For this review, take the finished solid that the model builds, in its own axes (mm). Face numbers are marked on the shaded views. A direction names the side the tool comes from. Coordinates: 2 decimals unless noted, no trailing zeros. Use a Markdown table: item, result.
from build123d import *

# Parameters (mm, degrees)
BASPROSKE_W        = 30
BASPROSKE_H        = 50
TOOTHCUT_DEPTH     = 77.811457479
TEETHCUTS_COUNT    = 23
TEETHCUTS_ANGLE    = 344.347826087
HUBNEABOTSKE_R     = 20
HUBNEARBOTH_DEPTH  = 5.0000254
HUBFAR_START       = 5.0000254
HUBFARSKE_R        = 20
HUBFAR_DEPTH       = 5.0000254
BORSKE_R           = 12
BORE_DEPTH         = 40.0000508
KEYSKE_W           = 8
KEYSKE_H           = 15.3
KEYWAY_DEPTH       = 40.0000508
SKETCH1_R          = 35
SKETCH1_R_2        = 20
CUT_EXTRUDE1_DEPTH = 14
FILLET1_R          = 4
CUT_EXTRUDE2_START = -14
SKETCH2_R          = 35
SKETCH2_R_2        = 20
CUT_EXTRUDE2_DEPTH = 14
FILLET2_R          = 4


with BuildPart() as part:
    # BasProSke → Base-Revolve (revolve)
    with BuildSketch(Plane(origin=(0, 0, 0), x_dir=(1, 0, 0), z_dir=(0, 1, 0)), mode=Mode.PRIVATE) as base_revolve_sk:
        with Locations((15, 25)):
            Rectangle(BASPROSKE_W, BASPROSKE_H)
    revolve(base_revolve_sk.sketch.rotate(Axis((-10, 0, 0), (1, 0, 0)), 180), axis=Axis((-10, 0, 0), (1, 0, 0)))

    # TooCutSke → ToothCut (cut, through all)
    with BuildSketch(Plane(origin=(0, 0, 0), x_dir=(0, 0, -1), z_dir=(1, 0, 0))):
        with BuildLine():
            ThreePointArc((1.90971626, 40.954498957), (0, 40.999), (-1.90971626, 40.954498957))
            ThreePointArc((-1.90971626, 40.954498957), (-3.228022445, 45.57670564), (-5.698439072, 49.699783071))
            ThreePointArc((-5.698439072, 49.699783071), (0, 50.0254), (5.698439072, 49.699783071))
            ThreePointArc((5.698439072, 49.699783071), (3.228022445, 45.57670564), (1.90971626, 40.954498957))
        make_face()
    toothcut = extrude(amount=TOOTHCUT_DEPTH, mode=Mode.SUBTRACT)

    # TeethCuts: ToothCut ×23 about axis
    teethcuts_axis = Axis((-10, 0, 0), (1, 0, 0))
    for i in range(1, TEETHCUTS_COUNT):
        add(toothcut.rotate(teethcuts_axis, i * TEETHCUTS_ANGLE / (TEETHCUTS_COUNT - 1)), mode=Mode.SUBTRACT)

    # HubNeaBotSke → HubNearBoth (add)
    with BuildSketch(Plane.ZY):
        with Locations(Location((0, 0, 0), (0, 0, 180))):
            Circle(HUBNEABOTSKE_R)
    extrude(amount=HUBNEARBOTH_DEPTH)

    # HubFarSke → HubFar (add)
    with BuildSketch(Plane(origin=(30, 0, 0), x_dir=(0, 0, -1), z_dir=(1, 0, 0)).offset(HUBFAR_START)):
        Circle(HUBFARSKE_R)
    extrude(amount=-HUBFAR_DEPTH)

    # BorSke → Bore (cut, symmetric)
    with BuildSketch(Plane(origin=(0, 0, 0), x_dir=(0, 0, -1), z_dir=(1, 0, 0))):
        with Locations(Location((0, 0, 0), (0, 0, 180))):
            Circle(BORSKE_R)
    extrude(amount=BORE_DEPTH, both=True, mode=Mode.SUBTRACT)

    # KeySke → Keyway (cut, symmetric)
    with BuildSketch(Plane(origin=(0, 0, 0), x_dir=(0, 0, -1), z_dir=(1, 0, 0))):
        with Locations((0, 7.65)):
            Rectangle(KEYSKE_W, KEYSKE_H)
    extrude(amount=KEYWAY_DEPTH, both=True, mode=Mode.SUBTRACT)

    # Sketch1 → Cut-Extrude1 (cut)
    with BuildSketch(Plane(origin=(30, 0, 0), x_dir=(0, 0, -1), z_dir=(1, 0, 0))):
        with Locations((0, 0.98088297)):
            Circle(SKETCH1_R)
        Circle(SKETCH1_R_2, mode=Mode.SUBTRACT)
    extrude(amount=-CUT_EXTRUDE1_DEPTH, mode=Mode.SUBTRACT)

    # Fillet1
    fillet1_edges = [part.edges().sort_by_distance(p)[0] for p in [
        (16, 0.98088297, 35),
        (16, 0, 20),
    ]]
    fillet(fillet1_edges, radius=FILLET1_R)

    # Sketch2 → Cut-Extrude2 (cut)
    with BuildSketch(Plane.ZY.offset(CUT_EXTRUDE2_START)):
        Circle(SKETCH2_R)
        Circle(SKETCH2_R_2, mode=Mode.SUBTRACT)
    extrude(amount=CUT_EXTRUDE2_DEPTH, mode=Mode.SUBTRACT)

    # Fillet2
    # the kernel refuses this fillet: 4 mm, written as the material it adds along each edge
    with BuildSketch(Plane(origin=(14, 0, 0), x_dir=(0, 0, 1), z_dir=(0, -1, 0))) as fillet2_piece_1:
        with BuildLine():
            CenterArc((35 - FILLET2_R, FILLET2_R), FILLET2_R, 270, 90)
            Line((35, FILLET2_R), (35, 0))
            Line((35, 0), (35 - FILLET2_R, 0))
        make_face()
    revolve(axis=Axis((14, 0, 0), (-1, 0, 0)))
    with BuildSketch(Plane(origin=(14, 0, 0), x_dir=(0, 0, 1), z_dir=(0, -1, 0))) as fillet2_piece_2:
        with BuildLine():
            CenterArc((20 + FILLET2_R, FILLET2_R), FILLET2_R, 180, 90)
            Line((20 + FILLET2_R, 0), (20, 0))
            Line((20, 0), (20, FILLET2_R))
        make_face()
    revolve(axis=Axis((14, 0, 0), (-1, 0, 0)))


solid = part.part
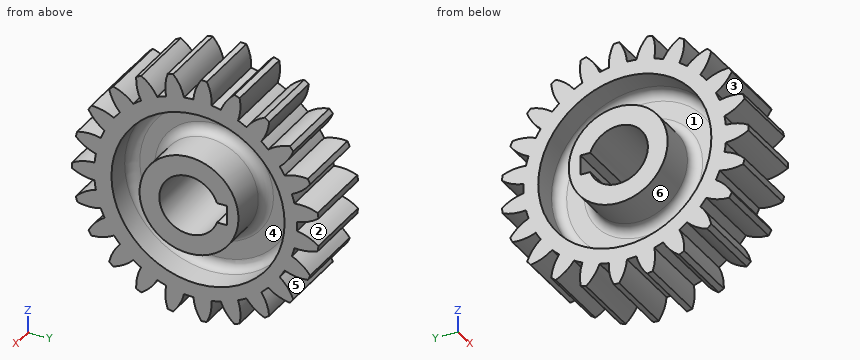
(1) Mouldability with a two-part tool opening along Y and no side actions: class the marked faces 1, 2 and 3 as pulls with the +Y half, pulls with the -Y half, needs draft (parallel to the pull), parting line crosses it, or undercut.
Found:
| item | result |
|---|---|
| face 1 | undercut |
| face 2 | pulls with the +Y half |
| face 3 | pulls with the -Y half |
(2) For pin 1 Ø5 at (x, y) = (0, -33) entering from -Z; pin 2 Ø3 at (x, y) = (11.5, 13.5) entering from -Z; pin 3 Ø2 at (x, z) = (6, -17) entering from -Y, all flat-tipped, find the tip position at first contact; note any pin that passes through.
Found:
| item | result |
|---|---|
| pin 1 | stops at z = -37.31 |
| pin 2 | stops at z = -46.89 |
| pin 3 | stops at y = -37.75 |
(3) Take a section at A-A on x = 27.5. State how many separate pieces and enclosed holes the cut face has, plus the area to 3 significant figures.
Found:
| item | result |
|---|---|
| separate pieces | 2 |
| enclosed holes | 2 |
| area | 3,390 mm^2 |
(4) For the marked faces 4, 5 and 6, list the 3-axis set-ups (+Z, -Z, +X, -X, +Y, -Y) from which the entire face can be reached by the end or side of a thin tool; tool diameter is ignored.
Found:
| item | result |
|---|---|
| face 4 | +X |
| face 5 | +X, -X, +Y |
| face 6 | -X |
(5) For line 1 along Y through (x, z) = (9, -30.5); line 2 along Z through (x, y) = (10, 13); line 3 along Z through (x, y) = (12, 13), list the stretches that pass through material, from the lowest coordinate up.
Found:
| item | result |
|---|---|
| line 1 | y = -32.9 to -17.17, 17.17 to 27.4, 32.21 to 39.43 |
| line 2 | z = -44.73 to -32.5, -15.2 to -4, 4 to 15.2, 32.5 to 44.73 |
| line 3 | z = -44.73 to -31.92, -15.9 to -4, 4 to 15.9, 31.92 to 44.73 |
